Work out the finished part from the listing and answer in its coordinate system (mm). A direction names the side the tool comes from. Round coordinates to 2 decimals unless told otherwise and drop trailing zeros. Loops run counter-clockwise (first coordinate to the right, second up) from the corner with the lowest first, then second, coordinate; pieces in that order, holes last. Notation, with made-up numbers: M 35.25,-22 L 78.25,-22 A25 ccw 78.25,3 Z; hole C 54.25,80.25 d8. An arc over 180 degrees is marked long. One line per item, written item: value.
```python
from build123d import *

# Parameters (mm, degrees)
SKETCH1_W                 = 150
SKETCH1_H                 = 200
BOSS_EXTRUDE1_DEPTH       = 2
SKETCH2_W                 = 6
SKETCH2_H                 = 10
SKETCH2_W_2               = 10
SKETCH2_H_2               = 6
CUT_EXTRUDE1_DEPTH        = 126.015998976
SKETCH5_W                 = 146
SKETCH5_H                 = 196
BOSS_EXTRUDE2_DEPTH       = 10
SKETCH6_W                 = 27.2
SKETCH6_H                 = 10
CUT_EXTRUDE2_DEPTH        = 10
SKETCH8_R                 = 1.7
CUT_EXTRUDE4_DEPTH        = 181.676506497
SKETCH10_W                = 20
SKETCH10_H                = 10
CUT_EXTRUDE6_DEPTH        = 10
SKETCH15_R                = 1.7
CUT_EXTRUDE7_DEPTH        = 10
SKETCH16_R                = 1.7
CUT_EXTRUDE8_DEPTH        = 3
SKETCH19_R                = 4
BOSS_EXTRUDE3_DEPTH       = 5
SKETCH20_R                = 2.6
CUT_EXTRUDE10_DEPTH       = 5
BOSS_EXTRUDE4_DEPTH       = 3
SKETCH22_W                = 2
SKETCH22_H                = 20
BOSS_EXTRUDE5_DEPTH       = 48
SKETCH25_W                = 0.5
SKETCH25_H                = 5
CUT_EXTRUDE13_DEPTH       = 58
SKETCH26_R                = 1.7
CUT_EXTRUDE15_DEPTH       = 5
SKETCH27_W                = 20
SKETCH27_H                = 20
BOSS_EXTRUDE6_DEPTH       = 5
BOSS_EXTRUDE7_DEPTH       = 20
SKETCH29_R                = 4
CUT_EXTRUDE16_DEPTH       = 10
SKETCH31_R                = 1.7
CUT_EXTRUDE17_DEPTH       = 179.395627749
BOSS_EXTRUDE9_DEPTH       = 3
SKETCH35_W                = 15.5
SKETCH35_H                = 15.5
BOSS_EXTRUDE10_DEPTH      = 58
SKETCH36_R                = 2.6
CUT_EXTRUDE20_DEPTH       = 5
SKETCH38_R                = 2.6
CUT_EXTRUDE21_DEPTH       = 5
SKETCH37_W                = 4
SKETCH37_H                = 15
BOSS_EXTRUDE11_DEPTH      = 45.92
BOSS_EXTRUDE12_DEPTH      = 4
BOSS_EXTRUDE12_DEPTH_BACK = 4
FILLET1_R                 = 100
BOSS_EXTRUDE13_DEPTH      = 8
FILLET2_R                 = 100
SKETCH41_R                = 2.6
CUT_EXTRUDE22_DEPTH       = 5
SKETCH42_W                = 99.5
SKETCH42_H                = 33
CUT_EXTRUDE23_DEPTH       = 1


with BuildPart() as part:
    # Sketch1 → Boss-Extrude1 (new body)
    with BuildSketch(Plane(origin=(0, 0, 0), x_dir=(1, 0, 0), z_dir=(0, 1, 0))):
        Rectangle(SKETCH1_W, SKETCH1_H)
    extrude(amount=BOSS_EXTRUDE1_DEPTH)

    # Sketch2 → Cut-Extrude1 (cut, through all)
    with BuildSketch(Plane(origin=(0, 2, 0), x_dir=(1, 0, 0), z_dir=(0, 1, 0))):
        with Locations((-65, 5)):
            Rectangle(SKETCH2_W, SKETCH2_H)
        with Locations((17.5, -90)):
            Rectangle(SKETCH2_W_2, SKETCH2_H_2)
        with Locations((-40.588652837, 90)):
            Rectangle(SKETCH2_W_2, SKETCH2_H_2)
    extrude(amount=-CUT_EXTRUDE1_DEPTH, mode=Mode.SUBTRACT)

    # Sketch5 → Boss-Extrude2 (add)
    with BuildSketch(Plane(origin=(0, 2, 0), x_dir=(1, 0, 0), z_dir=(0, 1, 0))):
        Polygon((-75, 100), (-75, -100), (75, -100), (75, -98), (75, 98), (75, 100), align=None)
        Rectangle(SKETCH5_W, SKETCH5_H, mode=Mode.SUBTRACT)
    extrude(amount=BOSS_EXTRUDE2_DEPTH)

    # Sketch6 → Cut-Extrude2 (cut)
    with BuildSketch(Plane.ZY.offset(75)):
        with Locations((-64.4, 7)):
            Rectangle(SKETCH6_W, SKETCH6_H)
    extrude(amount=-CUT_EXTRUDE2_DEPTH, mode=Mode.SUBTRACT)

    # Sketch8 → Cut-Extrude4 (cut, through all)
    with BuildSketch(Plane.ZY.offset(75)):
        with Locations((5, 7)):
            Circle(SKETCH8_R)
    extrude(amount=-CUT_EXTRUDE4_DEPTH, mode=Mode.SUBTRACT)

    # Sketch10 → Cut-Extrude6 (cut)
    with BuildSketch(Plane(origin=(75, 0, 0), x_dir=(0, 0, -1), z_dir=(1, 0, 0))):
        with Locations((12, 7)):
            Rectangle(SKETCH10_W, SKETCH10_H)
    extrude(amount=-CUT_EXTRUDE6_DEPTH, mode=Mode.SUBTRACT)

    # Sketch15 → Cut-Extrude7 (cut)
    with BuildSketch(Plane.XY.offset(100)):
        with Locations((0, 7)):
            Circle(SKETCH15_R)
    extrude(amount=-CUT_EXTRUDE7_DEPTH, mode=Mode.SUBTRACT)

    # Sketch16 → Cut-Extrude8 (cut)
    with BuildSketch(Plane.XY.offset(100)):
        with Locations((67, 7)):
            Circle(SKETCH16_R)
    extrude(amount=-CUT_EXTRUDE8_DEPTH, mode=Mode.SUBTRACT)

    # Sketch19 → Boss-Extrude3 (add)
    with BuildSketch(Plane(origin=(0, 2, 0), x_dir=(1, 0, 0), z_dir=(0, 1, 0))):
        with Locations(Location((-60.85, -90, 0), (0, 0, 270))):
            Circle(SKETCH19_R)
        with Locations(Location((-11.85, -90, 0), (0, 0, 270))):
            Circle(SKETCH19_R)
        with Locations(Location((-45.23, -17.9, 0), (0, 0, 270))):
            Circle(SKETCH19_R)
        with Locations(Location((-17.32, -17.9, 0), (0, 0, 270))):
            Circle(SKETCH19_R)
    extrude(amount=BOSS_EXTRUDE3_DEPTH)

    # Sketch20 → Cut-Extrude10 (cut)
    with BuildSketch(Plane(origin=(0, 7, 0), x_dir=(1, 0, 0), z_dir=(0, 1, 0))):
        with Locations(Location((-45.23, -17.9, 0), (0, 0, 270))):
            Circle(SKETCH20_R)
        with Locations(Location((-17.32, -17.9, 0), (0, 0, 270))):
            Circle(SKETCH20_R)
        with Locations(Location((-11.85, -90, 0), (0, 0, 270))):
            Circle(SKETCH20_R)
        with Locations(Location((-60.85, -90, 0), (0, 0, 270))):
            Circle(SKETCH20_R)
    extrude(amount=-CUT_EXTRUDE10_DEPTH, mode=Mode.SUBTRACT)

    # Sketch21 → Boss-Extrude4 (add)
    with BuildSketch(Plane(origin=(0, 2, 0), x_dir=(1, 0, 0), z_dir=(0, 1, 0))):
        Polygon((-29.5, 65), (-32.5, 65), (-32.5, 59), (70, 59), (70, 62), (-29.5, 62), align=None)
    extrude(amount=BOSS_EXTRUDE4_DEPTH)

    # Sketch22 → Boss-Extrude5 (add)
    with BuildSketch(Plane(origin=(0, 12, 0), x_dir=(1, 0, 0), z_dir=(0, 1, 0))):
        with Locations((-74, 40.8)):
            Rectangle(SKETCH22_W, SKETCH22_H)
        Polygon((-75, 100), (-53, 100), (-53, 98), (-73, 98), (-73, 78), (-75, 78), align=None)
    extrude(amount=BOSS_EXTRUDE5_DEPTH)

    # Sketch25 → Cut-Extrude13 (cut)
    with BuildSketch(Plane(origin=(0, 60, 0), x_dir=(1, 0, 0), z_dir=(0, 1, 0))):
        with Locations((-73.25, 80.5)):
            Rectangle(SKETCH25_W, SKETCH25_H)
        with Locations((-73.25, 48.3)):
            Rectangle(SKETCH25_W, SKETCH25_H)
    extrude(amount=-CUT_EXTRUDE13_DEPTH, mode=Mode.SUBTRACT)

    # Sketch26 → Cut-Extrude15 (cut)
    with BuildSketch(Plane(origin=(75, 0, 0), x_dir=(0, 0, -1), z_dir=(1, 0, 0))):
        with Locations((88, 7)):
            Circle(SKETCH26_R)
    extrude(amount=-CUT_EXTRUDE15_DEPTH, mode=Mode.SUBTRACT)

    # Sketch27 → Boss-Extrude6 (add)
    with BuildSketch(Plane(origin=(0, 2, 0), x_dir=(1, 0, 0), z_dir=(0, 1, 0))):
        with Locations((-60, 40.8)):
            Rectangle(SKETCH27_W, SKETCH27_H)
    extrude(amount=BOSS_EXTRUDE6_DEPTH)

    # Sketch28 → Boss-Extrude7 (add)
    with BuildSketch(Plane.XY.offset(-30.8)):
        Polygon((-70, 7), (-70, 60), (-60, 60), (-50, 7), align=None)
    extrude(amount=-BOSS_EXTRUDE7_DEPTH)

    # Sketch29 → Cut-Extrude16 (cut)
    with BuildSketch(Plane(origin=(-50, 0, 0), x_dir=(0, 0, -1), z_dir=(1, 0, 0))):
        with Locations((40.087803788, 47)):
            Circle(SKETCH29_R)
    extrude(amount=-CUT_EXTRUDE16_DEPTH, mode=Mode.SUBTRACT)

    # Sketch31 → Cut-Extrude17 (cut, through all)
    with BuildSketch(Plane(origin=(-60, 0, 0), x_dir=(0, 0, -1), z_dir=(1, 0, 0))):
        with Locations((40.087803788, 47)):
            Circle(SKETCH31_R)
    extrude(amount=-CUT_EXTRUDE17_DEPTH, mode=Mode.SUBTRACT)

    # Sketch34 → Boss-Extrude9 (add)
    with BuildSketch(Plane(origin=(0, 2, 0), x_dir=(1, 0, 0), z_dir=(0, 1, 0))):
        Polygon((-4.5, 59), (-4.5, -24), (51.5, -24), (51.5, 59), (54.5, 59), (54.5, -27), (-7.5, -27), (-7.5, 59), align=None)
    extrude(amount=BOSS_EXTRUDE9_DEPTH)

    # Sketch35 → Boss-Extrude10 (add)
    with BuildSketch(Plane(origin=(0, 2, 0), x_dir=(1, 0, 0), z_dir=(0, 1, 0))):
        with Locations((62.25, 51.25)):
            Rectangle(SKETCH35_W, SKETCH35_H)
    extrude(amount=BOSS_EXTRUDE10_DEPTH)

    # Sketch36 → Cut-Extrude20 (cut)
    with BuildSketch(Plane(origin=(0, 60, 0), x_dir=(1, 0, 0), z_dir=(0, 1, 0))):
        with Locations(Location((62.25, 51.25, 0), (0, 0, 270))):
            Circle(SKETCH36_R)
    extrude(amount=-CUT_EXTRUDE20_DEPTH, mode=Mode.SUBTRACT)

    # Sketch38 → Cut-Extrude21 (cut)
    with BuildSketch(Plane(origin=(0, 60, 0), x_dir=(1, 0, 0), z_dir=(0, 1, 0))):
        with Locations(Location((-65, 40.8, 0), (0, 0, 270))):
            Circle(SKETCH38_R)
    extrude(amount=-CUT_EXTRUDE21_DEPTH, mode=Mode.SUBTRACT)

    # Sketch37 → Boss-Extrude11 (add)
    with BuildSketch(Plane(origin=(0, 2, 0), x_dir=(1, 0, 0), z_dir=(0, 1, 0))):
        with Locations((-68, -50.073123899)):
            Rectangle(SKETCH37_W, SKETCH37_H)
        with Locations((68, -50.073123899)):
            Rectangle(SKETCH37_W, SKETCH37_H)
    extrude(amount=BOSS_EXTRUDE11_DEPTH)

    # Sketch39 → Boss-Extrude12 (add, two sides: drawn at the far end of the back side and taken through both)
    with BuildSketch(Plane(origin=(-66, 0, 0), x_dir=(0, 0, -1), z_dir=(1, 0, 0)).offset(-BOSS_EXTRUDE12_DEPTH_BACK)):
        Polygon((-57.573123899, 47.92), (-42.573123899, 47.92), (-42.573123899, 51.89), align=None)
    extrude(amount=BOSS_EXTRUDE12_DEPTH + BOSS_EXTRUDE12_DEPTH_BACK)

    # Fillet1
    # the kernel refuses this fillet: 100 mm, written as the material it adds along each edge
    with BuildSketch(Plane(origin=(-66, 47.92, 57.573123899), x_dir=(1, 0, 0), z_dir=(0, 0, -1))) as fillet1_piece_1_section:
        with BuildLine():
            CenterArc((100, 28), FILLET1_R, 180, 16.260204708)
            Line((0, 28), (-2, 28))
            Line((-2, 28), (-2, 0))
            Line((-2, 0), (0, -2))
            ThreePointArc((0, -2), (2, -2), (2.08, -0.56))
            Line((2.08, -0.56), (4, 0))
        make_face()
    fillet1_piece_1 = extrude(amount=15, mode=Mode.PRIVATE)
    fillet1_piece_1 = split(fillet1_piece_1, bisect_by=Plane(origin=(-66.078013707, 49.109205827, 53.07990289), z_dir=(0, -0.9667146052036466, -0.25585713217723216)), keep=Keep.TOP, mode=Mode.PRIVATE)
    add(fillet1_piece_1)

    # Sketch40 → Boss-Extrude13 (add)
    with BuildSketch(Plane(origin=(70, 0, 0), x_dir=(0, 0, -1), z_dir=(1, 0, 0))):
        Polygon((-42.573123899, 47.92), (-42.573123899, 51.89), (-57.573123899, 47.92), align=None)
    extrude(amount=-BOSS_EXTRUDE13_DEPTH)

    # Fillet2
    # the kernel refuses this fillet: 100 mm, written as the material it adds along each edge
    with BuildSketch(Plane(origin=(66, 47.92, 42.573123899), x_dir=(-1, 0, 0), z_dir=(0, 0, 1))) as fillet2_piece_1_section:
        with BuildLine():
            CenterArc((100, 28), FILLET2_R, 180, 16.260204708)
            Line((0, 28), (-2, 28))
            Line((-2, 28), (-2, 0))
            Line((-2, 0), (0, -2))
            ThreePointArc((0, -2), (2, -2), (2.08, -0.56))
            Line((2.08, -0.56), (4, 0))
        make_face()
    fillet2_piece_1 = extrude(amount=15, mode=Mode.PRIVATE)
    fillet2_piece_1 = split(fillet2_piece_1, bisect_by=Plane(origin=(66.078013707, 49.109205827, 53.07990289), z_dir=(0, -0.9667146052036466, -0.25585713217723216)), keep=Keep.TOP, mode=Mode.PRIVATE)
    add(fillet2_piece_1)

    # Sketch41 → Cut-Extrude22 (cut)
    with BuildSketch(Plane(origin=(0, 59.02320322, 15.621474452), x_dir=(1, 0, 0), z_dir=(0, 0.9667146052036468, 0.2558571321772319))):
        with Locations(Location((-66, -35.63787002, 0), (0, 0, 270))):
            Circle(SKETCH41_R)
        with Locations(Location((66, -35.63787002, 0), (0, 0, 270))):
            Circle(SKETCH41_R)
    extrude(amount=-CUT_EXTRUDE22_DEPTH, mode=Mode.SUBTRACT)

    # Sketch42 → Cut-Extrude23 (cut)
    with BuildSketch(Plane(origin=(0, 2, 0), x_dir=(1, 0, 0), z_dir=(0, 1, 0))):
        with Locations((20.25, 78.5)):
            Rectangle(SKETCH42_W, SKETCH42_H)
    extrude(amount=-CUT_EXTRUDE23_DEPTH, mode=Mode.SUBTRACT)


solid = part.part
```
1) Find the intervals of material crossed by probe 1 along Z at (x, y) = (-68, 36); probe 2 along X at (y, z) = (4.5, -31.5); probe 3 along Z at (x, y) = (-45, 3), in increasing order. Write a range as from..to.
Check values:
probe 1: -100..-98, -50.8..-30.8, 42.57..57.57
probe 2: -75..-73, -70..-50, -7.5..-4.5, 51.5..54.5, 73..75
probe 3: -100..-98, 13.91..15.31, 20.49..21.89, 98..100
2) The mould has two halves that part along Y. Classify faces 1 (the face through (-63.42, 47.61, 49.12)), 2 (the face through (-66, 60, -38)), 3 (the face through (-73.5, 31, -48)): +Y half, -Y half, draft (parallel to the pull), parting line (faces both ways), or undercut.
Check values:
face 1: undercut
face 2: +Y half
face 3: draft
3) Find section B-B (x = 36). Give the vertices of the cut face in (y, z).
Check values:
outline: M 0,-100 L 12,-100 L 12,-98 L 2,-98 L 2,-95 L 1,-95 L 1,-62 L 5,-62 L 5,-59 L 2,-59 L 2,24 L 5,24 L 5,27 L 2,27 L 2,98 L 12,98 L 12,100 L 0,100 Z
4) For faces 4 (the face through (-62.422, 57.535, -41.138)), 5 (the face through (-62, 25, -50.8)), 6 (the face through (-58.7, 43.1, -39.2)), determine the directions among +Z, -Z, +X, -X, +Y, -Y from which every point of the face is accessible in a straight line to the end or side of a thin tool.
Check values:
face 4: +Y
face 5: -X, +Y
face 6: none
5) Find section A-A (z = 90). Give the vertices of the cut face in (x, y), then the cut area to 3 significant figures.
Check values:
outline: M -75,0 L 12.5,0 L 12.5,2 L -7.85,2 L -7.85,7 L -9.25,7 L -9.25,2 L -14.45,2 L -14.45,7 L -15.85,7 L -15.85,2 L -56.85,2 L -56.85,7 L -58.25,7 L -58.25,2 L -63.45,2 L -63.45,7 L -64.85,7 L -64.85,2 L -73,2 L -73,12 L -75,12 Z; M 22.5,0 L 75,0 L 75,12 L 73,12 L 73,2 L 22.5,2 Z
area: 348 mm2
6) Find section C-C (y = 24). Give the number of separate pieces and of enclosed holes in the cut face, then the cut area to 3 significant figures.
Check values:
separate pieces: 6
enclosed holes: 0
area: 818 mm2
7) Each of these flat-tipped pins is pushed along its axis until it touches: pin 1 (16.5 mm diameter, centred on x = 7.5, z = -81.5, fed in from +Y); pin 2 (2.5 mm diameter, centred on x = -18, z = 19, fed in from +Y); pin 3 (1 mm diameter, centred on y = 25.5, z = -99, fed in from +X). Where does it stop, or does it pass through?
Check values:
pin 1: y = 1
pin 2: y = 2
pin 3: x = -53
